from build123d import *

# Parameters (mm, degrees)
ESBO_O1_R                = 1.65
ESBO_O1_R_2              = 11.1
RESSALTO_EXTRUS_O1_DEPTH = 6
RESSALTO_EXTRUS_O2_DEPTH = 19
CHANFRO1_SIZE            = 10
CHANFRO2_SIZE            = 19
CORTE_EXTRUS_O1_REACH    = 46
ESBO_O3_R                = 2.65


with BuildPart() as part:
    # Esbo_o1 → Ressalto-extrus_o1 (new body)
    with BuildSketch(Plane.XY):
        Polygon((39.50000006, -17.500000656), (39.50000006, -22.500000656), (22.00000006, -22.500000656), (22.00000006, -42.500000656), (-21.99999994, -42.500000656), (-21.99999994, -22.500000656), (-39.49999994, -22.500000656), (-39.49999994, -17.500000656), (-26.99999994, -17.500000656), (-26.99999994, 1.499999344), (-21.99999994, 1.499999344), (-21.99999994, 21.499999344), (22.00000006, 21.499999344), (22.00000006, 1.499999344), (27.00000006, 1.499999344), (27.00000006, -17.500000656), align=None)
        with Locations((15.50000006, 15.499999344)):
            Circle(ESBO_O1_R, mode=Mode.SUBTRACT)
        with Locations((15.50000006, -15.500000656)):
            Circle(ESBO_O1_R, mode=Mode.SUBTRACT)
        with Locations((-15.49999994, 15.499999344)):
            Circle(ESBO_O1_R, mode=Mode.SUBTRACT)
        with Locations((-15.49999994, -15.500000656)):
            Circle(ESBO_O1_R, mode=Mode.SUBTRACT)
        Circle(ESBO_O1_R_2, mode=Mode.SUBTRACT)
        with BuildLine():
            Line((-4.99999994, -35.250000656), (-4.99999994, -35.750000656))
            Line((-4.99999994, -35.750000656), (5.00000006, -35.750000656))
            Line((5.00000006, -35.750000656), (5.00000006, -35.250000656))
            Line((5.00000006, -35.250000656), (11.00000006, -35.250000656))
            ThreePointArc((11.00000006, -35.250000656), (13.75000006, -32.500000656), (11.00000006, -29.750000656))
            Line((11.00000006, -29.750000656), (5.00000006, -29.750000656))
            Line((5.00000006, -29.750000656), (5.00000006, -29.250000656))
            Line((5.00000006, -29.250000656), (-4.99999994, -29.250000656))
            Line((-4.99999994, -29.250000656), (-4.99999994, -29.750000656))
            Line((-4.99999994, -29.750000656), (-10.99999994, -29.750000656))
            ThreePointArc((-10.99999994, -29.750000656), (-13.74999994, -32.500000656), (-10.99999994, -35.250000656))
            Line((-10.99999994, -35.250000656), (-4.99999994, -35.250000656))
        make_face(mode=Mode.SUBTRACT)
    extrude(amount=RESSALTO_EXTRUS_O1_DEPTH)

    # Esbo_o2 → Ressalto-extrus_o2 (add)
    with BuildSketch(Plane.XY.offset(6)):
        Polygon((39.50000006, -22.500000656), (39.50000006, -17.500000656), (27.00000006, -17.500000656), (27.00000006, 1.499999344), (22.00000006, 1.499999344), (22.00000006, -22.500000656), align=None)
        Polygon((-39.49999994, -22.500000656), (-21.99999994, -22.500000656), (-21.99999994, 1.499999344), (-26.99999994, 1.499999344), (-26.99999994, -17.500000656), (-39.49999994, -17.500000656), align=None)
    extrude(amount=RESSALTO_EXTRUS_O2_DEPTH)

    # Chanfro1
    chanfro1_edges = [part.edges().sort_by_distance(p)[0] for p in [
        (39.50000006, -20.000000656, 25),
        (-39.49999994, -20.000000656, 25),
    ]]
    chamfer(chanfro1_edges, length=CHANFRO1_SIZE)

    # Chanfro2
    chanfro2_edges = [part.edges().sort_by_distance(p)[0] for p in [
        (-24.49999994, 1.499999344, 25),
        (24.50000006, 1.499999344, 25),
    ]]
    chamfer(chanfro2_edges, length=CHANFRO2_SIZE)

    # Esbo_o3 → Corte-extrus_o1 (cut, up to next)
    with BuildSketch(Plane.XZ.offset(22.500000656), mode=Mode.PRIVATE) as corte_extrus_o1_sk1:
        with Locations((32.50000006, 15.13)):
            Circle(ESBO_O3_R)
    corte_extrus_o1_tool1 = extrude(corte_extrus_o1_sk1.sketch, amount=-CORTE_EXTRUS_O1_REACH, mode=Mode.PRIVATE) & part.part
    add(corte_extrus_o1_tool1.solids().sort_by_distance((32.5, -22.500001, 15.13))[0], mode=Mode.SUBTRACT)
    # Esbo_o3 → Corte-extrus_o1 (cut, up to next)
    with BuildSketch(Plane.XZ.offset(22.500000656), mode=Mode.PRIVATE) as corte_extrus_o1_sk2:
        with Locations((-32.49999994, 15.13)):
            Circle(ESBO_O3_R)
    corte_extrus_o1_tool2 = extrude(corte_extrus_o1_sk2.sketch, amount=-CORTE_EXTRUS_O1_REACH, mode=Mode.PRIVATE) & part.part
    add(corte_extrus_o1_tool2.solids().sort_by_distance((-32.5, -22.500001, 15.13))[0], mode=Mode.SUBTRACT)


solid = part.part
Build history of the part. All positions in model axes, mm. A direction names the side the tool comes from. Coordinates: 2 decimals unless noted, no trailing zeros. Write each loop counter-clockwise with the first axis right and the second up, starting at its lowest first coordinate (ties: lowest second). Pieces come first, ordered by that corner, then holes.
(1) Mould opens along Y. For faces 5 (the cylindrical face through (16.261, -16.964, 2.958)), 6 (the flat face through (31, -22.5, 12)), 7 (the cylindrical face through (-32.84, -20.04, 17.76)), 8 (the flat face through (8, -35.25, 3)) say: pulls with the +Y half, pulls with the -Y half, needs draft (parallel to the pull), parting line crosses it, or undercut.
(2) Cut at A-A on x = 32.5. List the corners of the cut face in (y, z).
(3) Pin check, flat tips, straight feed: pin 1 Ø6 at (y, z) = (2.5, 9) entering from +X; pin 2 Ø1 at (x, y) = (8, 7.5) entering from +Z; pin 3 Ø1.5 at (x, z) = (-27, 4.5) entering from +Y. Stop position of each tip, or through.
(4) 3-axis set-ups, long thin cutter, end or side, ignore diameter. For faces 1 (the flat face through (22, -32, 3)), 2 (the flat face through (-22, 11, 3)), 3 (the flat face through (-31, -22.5, 12)), 4 (the cylindrical face through (13.75, -32.56, 2.96)): which of +Z, -Z, +X, -X, +Y, -Y reach the whole face in a straight line?
(5) Cut at D-D on y = 15.5. List the corners of the cut face in (x, z), and give its area (3 significant figures).
(6) Cut at C-C on x = 0. List the corners of the cut face in (y, z).
(7) Cut at B-B on y = -32.5. List the corners of the cut face in (x, z).
(8) Drill centre lines: line 1 (X direction, y = 15.5, z = 1.35); line 2 (Y direction, x = 15.5, z = 2.95); line 3 (Z direction, x = 32.5, y = -20.85). Where is each one in solid material? Low to high.
Working result:
1. face 5: undercut
1. face 6: pulls with the -Y half
1. face 7: needs draft
1. face 8: undercut
2. outline: (-22.5, 0) - (-17.5, 0) - (-17.5, 12.48) - (-22.5, 12.48) - close; (-22.5, 17.78) - (-17.5, 17.78) - (-17.5, 22) - (-22.5, 22) - close
3. pin 1: stops at x = 27
3. pin 2: stops at z = 6
3. pin 3: stops at y = 1.5
4. face 1: +Z, -Z, +X, -Y
4. face 2: +Z, -Z, -X, +Y
4. face 3: +Z, -Z, -X, -Y
4. face 4: +Z, -Z
5. outline: (-22, 0) - (-17.15, 0) - (-17.15, 6) - (-22, 6) - close; (-13.85, 0) - (13.85, 0) - (13.85, 6) - (-13.85, 6) - close; (17.15, 0) - (22, 0) - (22, 6) - (17.15, 6) - close
5. area: 224 mm2
6. outline: (-42.5, 0) - (-35.75, 0) - (-35.75, 6) - (-42.5, 6) - close; (-29.25, 0) - (-11.1, 0) - (-11.1, 6) - (-29.25, 6) - close; (11.1, 0) - (21.5, 0) - (21.5, 6) - (11.1, 6) - close
7. outline: (-22, 0) - (-13.75, 0) - (-13.75, 6) - (-22, 6) - close; (13.75, 0) - (22, 0) - (22, 6) - (13.75, 6) - close
8. line 1: x = -22 to -17.15, -13.85 to 13.85, 17.15 to 22
8. line 2: y = -42.5 to -17.15, -13.85 to 13.85, 17.15 to 21.5
8. line 3: z = 0 to 12.48, 17.78 to 22
